Check sheet for the modelled part. Datum: model origin and axes. Units: mm. A direction names the side the tool comes from. Give positions to 0.01 mm unless a question says otherwise; leave off trailing zeros. Order: outer loops, then holes, each group sorted by start corner. A loop starts at its lowest first (then second) coordinate and runs counter-clockwise, first axis right, second up. Notation, with made-up numbers: M -28,61.25 L 7,61.25 A16 cw 7,92.25 Z; hole C 86.25,48 d9. An arc over 180 degrees is marked long. Return JSON: item names as keys, results as strings. Group by question number.
from build123d import *

# Parameters (mm, degrees)
SKETCH1_W           = 72.136
SKETCH1_H           = 145.796
BOSS_EXTRUDE1_DEPTH = 5.207
FILLET1_R           = 2.54
SKETCH2_R           = 6.35
SKETCH2_R_2         = 1.905
SKETCH2_W           = 64.77
SKETCH2_H           = 105.56555142
CUT_EXTRUDE1_DEPTH  = 0.508
SKETCH4_R           = 3.81
CUT_EXTRUDE2_DEPTH  = 0.508
CUT_EXTRUDE3_DEPTH  = 0.508


with BuildPart() as part:
    # Sketch1 → Boss-Extrude1 (new, symmetric)
    with BuildSketch(Plane.XY):
        Rectangle(SKETCH1_W, SKETCH1_H)
    extrude(amount=BOSS_EXTRUDE1_DEPTH, both=True)

    # Fillet1
    fillet1_edges = [part.edges().sort_by_distance(p)[0] for p in [
        (36.068, -72.898, 0),
        (-36.068, -72.898, 0),
        (-36.068, 72.898, 0),
        (36.068, 72.898, 0),
    ]]
    fillet(fillet1_edges, radius=FILLET1_R)

    # Sketch2 → Cut-Extrude1 (cut)
    with BuildSketch(Plane.XY.offset(5.207)):
        with Locations((0, -62.94277571)):
            Circle(SKETCH2_R)
        with Locations((0, 67.920387855)):
            Circle(SKETCH2_R_2)
        Rectangle(SKETCH2_W, SKETCH2_H)
        with BuildLine():
            Line((-8.89, 64.110387855), (8.89, 64.110387855))
            ThreePointArc((8.89, 64.110387855), (10.16, 62.840387855), (8.89, 61.570387855))
            Line((8.89, 61.570387855), (-8.89, 61.570387855))
            ThreePointArc((-8.89, 61.570387855), (-10.16, 62.840387855), (-8.89, 64.110387855))
        make_face()
    extrude(amount=-CUT_EXTRUDE1_DEPTH, mode=Mode.SUBTRACT)

    # Sketch4 → Cut-Extrude2 (cut)
    with BuildSketch(Plane(origin=(0, 0, -5.207), x_dir=(-1, 0, 0), z_dir=(0, 0, -1))):
        with Locations((25.4, 63.5)):
            Circle(SKETCH4_R)
    extrude(amount=-CUT_EXTRUDE2_DEPTH, mode=Mode.SUBTRACT)

    # Sketch5 → Cut-Extrude3 (cut)
    with BuildSketch(Plane(origin=(36.068, 0, 0), x_dir=(0, 0, -1), z_dir=(1, 0, 0))):
        with BuildLine():
            Line((1.27, 54.61), (1.27, 46.99))
            ThreePointArc((1.27, 46.99), (0, 45.72), (-1.27, 46.99))
            Line((-1.27, 46.99), (-1.27, 54.61))
            ThreePointArc((-1.27, 54.61), (0, 55.88), (1.27, 54.61))
        make_face()
        with BuildLine():
            Line((1.27, 41.91), (1.27, 34.29))
            ThreePointArc((1.27, 34.29), (0, 33.02), (-1.27, 34.29))
            Line((-1.27, 34.29), (-1.27, 41.91))
            ThreePointArc((-1.27, 41.91), (0, 43.18), (1.27, 41.91))
        make_face()
    extrude(amount=-CUT_EXTRUDE3_DEPTH, mode=Mode.SUBTRACT)


solid = part.part
1) Depth check by flat-ended pin: P1, Ø1.3, axis at y = 39.5, z = -0.5, coming from the +X side; P2, Ø1.1, axis at x = 0, y = 67.5, coming from the +Z side. Enter the tip coordinate at first touch or a pass-through.
2) Sectioned sample at B-B on y = 39. Record the boundary of the cut face in (x, z) (3 decimals).
3) Sectioned sample at D-D on y = 10. Record the boundary of the cut face in (x, z) (3 decimals), then the cut area to 3 significant figures.
4) Release check for a two-part mould opening along X. For faces 1 (the face through (0, -63, 4.699)), 2 (the face through (0, 72.898, 0)), 3 (the face through (35.344, -72.134, 0.073)) record: released by +X, released by -X, zero draft, split by the parting line, or undercut.
5) Material ranges on line 1 along Y through (x, z) = (0, 4.85); line 2 along Y through (x, z) = (-25.4, -4.95); line 3 along Z through (x, y) = (25.5, 52), recorded low to high.
6) Sectioned sample at A-A on x = 13.5. Record the boundary of the cut face in (y, z).
7) Tool access check on faces 4 (the face through (35.56, 38, 0)), 5 (the face through (-24.57, 59.78, -4.96)), 6 (the face through (-0.41, 66.06, 4.96)). Record the directions out of +Z, -Z, +X, -X, +Y, -Y that give a thin tool (end or side, any length) a straight path to the whole face; none if there is none.
8) Sectioned sample at C-C on x = -4.5. Record the boundary of the cut face in (y, z), then the cut area to 3 significant figures.
Reply:
{
 "1": {"P1": "x = 35.56", "P2": "z = 4.7"},
 "2": {"outline": "M -36.068,-5.207 L 36.068,-5.207 L 36.068,-1.27 L 35.56,-1.27 L 35.56,1.27 L 36.068,1.27 L 36.068,5.207 L 32.385,5.207 L 32.385,4.699 L -32.385,4.699 L -32.385,5.207 L -36.068,5.207 Z"},
 "3": {"outline": "M -36.068,-5.207 L 36.068,-5.207 L 36.068,5.207 L 32.385,5.207 L 32.385,4.699 L -32.385,4.699 L -32.385,5.207 L -36.068,5.207 Z", "area": "718 mm^2"},
 "4": {"face 1": "undercut", "face 2": "zero draft", "face 3": "released by +X"},
 "5": {"line 1": "-72.9 to -69.29, -56.59 to -52.78, 52.78 to 61.57, 64.11 to 66.02, 69.83 to 72.9", "line 2": "-72.9 to 59.69, 67.31 to 72.9", "line 3": "-5.21 to 4.7"},
 "6": {"outline": "M -72.9,-5.21 L 72.9,-5.21 L 72.9,5.21 L 52.78,5.21 L 52.78,4.7 L -52.78,4.7 L -52.78,5.21 L -72.9,5.21 Z"},
 "7": {"face 4": "+X", "face 5": "-Z", "face 6": "+Z"},
 "8": {"outline": "M -72.9,-5.21 L 72.9,-5.21 L 72.9,5.21 L 64.11,5.21 L 64.11,4.7 L 61.57,4.7 L 61.57,5.21 L 52.78,5.21 L 52.78,4.7 L -52.78,4.7 L -52.78,5.21 L -58.46,5.21 L -58.46,4.7 L -67.42,4.7 L -67.42,5.21 L -72.9,5.21 Z", "area": "1,460 mm^2"}
}
